Geometry: final body of the model. Coordinates: model frame, mm. Round coordinates to 2 decimals unless told otherwise and drop trailing zeros. Order: outer loops, then holes, each group sorted by start corner. A loop starts at its lowest first (then second) coordinate and runs counter-clockwise, first axis right, second up. Notation, with made-up numbers: (33, 82) - (92, 82) arc R15 cw to (92, 101) - close; hole circle Ø10 at (2, -39.75). An arc over 180 degrees is marked (long way). Put each result on its own line as item: value. Start each with the question number.
(1) Pin query (flat end, axial travel): P1, Ø3, axis at x = 81.28, y = 5.08, coming from the -Z side. Return the tip coordinate at first contact, or that it passes through.
(2) Material intervals for L1, parallel to Y at x = -81.28, z = 1.95; L2, parallel to X at y = 3.75, z = 2.4; L3, parallel to X at y = 2, z = 1.8, sorted ascending. Write a range as [from, to].
(3) Pull-direction query (X, two-part tool) for faces 1 (the face through (86.157, 10, 3)), 2 (the face through (-86.157, 10, 3)), 3 (the face through (83.626, 4.107, 2.576)); classes: released by +X, released by -X, zero draft, split by the parting line, or undercut.
(4) Section A-A (z = 4). Output: boundary loops of the cut face in (x, y), and give its area (3 significant figures).
from build123d import *

# Parameters (mm, degrees)
F1_DEPTH = 5.08
F2_R     = 2.54
F3_DEPTH = 5.081


with BuildPart() as f1:
    # F0 (on Top) → F1 (new body)
    with BuildSketch(Plane.XY):
        with BuildLine():
            Line((86.1568, 15.0368), (-86.1568, 15.0368))
            Line((-86.1568, 15.0368), (-86.1568, 5.08))
            ThreePointArc((-86.1568, 5.08), (-84.728418, 1.631582), (-81.28, 0.2032))
            Line((-81.28, 0.2032), (81.28, 0.2032))
            ThreePointArc((81.28, 0.2032), (84.728418, 1.631582), (86.1568, 5.08))
            Line((86.1568, 5.08), (86.1568, 15.0368))
        make_face()
    extrude(amount=F1_DEPTH)

    # F2 (on face) → F3 (cut, through all)
    with BuildSketch(Plane.XY.offset(5.08)):
        with Locations((-81.28, 5.08)):
            Circle(F2_R)
        with Locations((81.28, 5.08)):
            Circle(F2_R)
    extrude(amount=-F3_DEPTH, mode=Mode.SUBTRACT)


solid = f1.part
Checks:
1. P1: passes through
2. L1: y = [0.2, 2.54], [7.62, 15.04]
2. L2: x = [-85.97, -83.44], [-79.12, 79.12], [83.44, 85.97]
2. L3: x = [-85.06, 85.06]
3. face 1: released by +X
3. face 2: released by -X
3. face 3: undercut
4. outline: (-86.16, 5.08) arc R4.88 ccw to (-81.28, 0.2) - (81.28, 0.2) arc R4.88 ccw to (86.16, 5.08) - (86.16, 15.04) - (-86.16, 15.04) - close; hole circle Ø5.08 at (-81.28, 5.08); hole circle Ø5.08 at (81.28, 5.08)
4. area: 2,510 mm²
